```python
from build123d import *

# Parameters (mm, degrees)
BOSS_EXTRUDE1_DEPTH = 2.5
SKETCH1_5_W         = 50
SKETCH1_5_H         = 4.999999906
BOSS_EXTRUDE2_DEPTH = 2.5
SKETCH1_6_W         = 50
SKETCH1_6_H         = 1.524
SKETCH1_6_W_2       = 1.524
SKETCH1_6_H_2       = 25
BOSS_EXTRUDE3_DEPTH = 10


with BuildPart() as part:
    # Sketch1 → Boss-Extrude1 (new body)
    with BuildSketch(Plane(origin=(0, 0, 0), x_dir=(1, 0, 0), z_dir=(0, 1, 0))):
        Polygon((2.521, -2.499999953), (-2.521, -2.499999953), (-2.521, -4.023999953), (-2.521, -29.023999953), (2.521, -29.023999953), (2.521, -4.023999953), align=None)
    extrude(amount=BOSS_EXTRUDE1_DEPTH)

    # Sketch1_5 → Boss-Extrude2 (add)
    with BuildSketch(Plane(origin=(0, 0, 0), x_dir=(1, 0, 0), z_dir=(0, 1, 0))):
        Rectangle(SKETCH1_5_W, SKETCH1_5_H)
    extrude(amount=BOSS_EXTRUDE2_DEPTH)

    # Sketch1_6 → Boss-Extrude3 (add)
    with BuildSketch(Plane(origin=(0, 0, 0), x_dir=(1, 0, 0), z_dir=(0, 1, 0))):
        Polygon((25, -4.023999953), (25, -2.499999953), (2.521, -2.499999953), (2.521, -4.023999953), (4.045, -4.023999953), align=None)
        with Locations((0, 3.261999953)):
            Rectangle(SKETCH1_6_W, SKETCH1_6_H)
        with Locations((3.283, -16.523999953)):
            Rectangle(SKETCH1_6_W_2, SKETCH1_6_H_2)
        with Locations((-3.283, -16.523999953)):
            Rectangle(SKETCH1_6_W_2, SKETCH1_6_H_2)
        Polygon((-2.521, -2.499999953), (-25, -2.499999953), (-25, -4.023999953), (-4.045, -4.023999953), (-2.521, -4.023999953), align=None)
    extrude(amount=BOSS_EXTRUDE3_DEPTH)


solid = part.part
```
Input: part model. Units: mm. Frame: model coordinates. A direction names the side the tool comes from. Give positions to 0.01 mm unless a question says otherwise; leave off trailing zeros. Order: outer loops, then holes, each group sorted by start corner. A loop starts at its lowest first (then second) coordinate and runs counter-clockwise, first axis right, second up. Notation, with made-up numbers: M -19,15 L -14,15 A18 ccw -14,25 Z; hole C 38.25,11.25 d5. An arc over 180 degrees is marked long. Return JSON: item names as keys, results as strings.
1) Section query B-B on x = -6.5. Output: boundary loops of the cut face in (y, z).
Taken from the geometry:
{"outline": "M 0,-4.02 L 10,-4.02 L 10,-2.5 L 2.5,-2.5 L 2.5,2.5 L 10,2.5 L 10,4.02 L 0,4.02 Z"}
2) Contact query for flat-ended pins moving along their axis: pin 1 (2 mm diameter, centred on y = 5.5, z = 20, fed in from -X) (3 decimals); pin 2 (3 mm diameter, centred on x = 15.5, y = 3, fed in from +Z); pin 3 (5 mm diameter, centred on y = 3, z = 12.5, fed in from +X) (3 decimals). Output: stop coordinate, or through.
Taken from the geometry:
{"pin 1": "stops at x = -4.045", "pin 2": "stops at z = 4.02", "pin 3": "stops at x = 4.045"}
3) Line query: L1, parallel to Z at x = 13.5, y = 6; L2, parallel to X at y = 6.5, z = 13.5 (3 decimals); L3, parallel to Z at x = -3, y = 3. Output: solid intervals per line, ascending. Write a range as [from, to].
Taken from the geometry:
{"L1": "z = [-4.02, -2.5], [2.5, 4.02]", "L2": "x = [-4.045, -2.521], [2.521, 4.045]", "L3": "z = [-4.02, -2.5], [2.5, 29.02]"}
4) Section query A-A on y = 3.25. Output: boundary loops of the cut face in (x, z) (3 decimals), and give its area (3 significant figures).
Taken from the geometry:
{"outline": "M -25,-4.024 L 25,-4.024 L 25,-2.5 L -25,-2.5 Z; M -25,2.5 L -2.521,2.5 L -2.521,29.024 L -4.045,29.024 L -4.045,4.024 L -25,4.024 Z; M 2.521,2.5 L 25,2.5 L 25,4.024 L 4.045,4.024 L 4.045,29.024 L 2.521,29.024 Z", "area": "221 mm2"}
5) Mould query, pull axis X, two halves, no side actions, for faces 1 (the face through (25, 2, 0)), 2 (the face through (3.7, 10, 9.8)), 3 (the face through (2.521, 6, 16)), 4 (the face through (0, 2.5, 6)). Classes: released by +X, released by -X, zero draft, split by the parting line, or undercut.
Taken from the geometry:
{"face 1": "released by +X", "face 2": "zero draft", "face 3": "undercut", "face 4": "undercut"}
6) Access query for faces 5 (the face through (14, 5, 4.024)), 6 (the face through (-2.521, 6, 16)), 7 (the face through (0, 6, -2.5)), 8 (the face through (-4.045, 5, 17)). Directions: +Z, -Z, +X, -X, +Y, -Y. A direction counts if a zero-diameter tool reaches every point of the face in a straight line with its end or side. Return the directions, or none.
Taken from the geometry:
{"face 5": "+Z, +X, +Y, -Y", "face 6": "+Z, +Y", "face 7": "+X, -X, +Y", "face 8": "+Z, -X, +Y, -Y"}
7) Section query D-D on z = -1. Output: boundary loops of the cut face in (x, y).
Taken from the geometry:
{"outline": "M -25,0 L 25,0 L 25,2.5 L -25,2.5 Z"}
8) Section query C-C on z = 20. Output: boundary loops of the cut face in (x, y) (3 decimals).
Taken from the geometry:
{"outline": "M -4.045,0 L 4.045,0 L 4.045,10 L 2.521,10 L 2.521,2.5 L -2.521,2.5 L -2.521,10 L -4.045,10 Z"}
